For this review, take the finished solid that the model builds, in its own axes (mm). Coordinates: 2 decimals unless noted, no trailing zeros. Write each loop counter-clockwise with the first axis right and the second up, starting at its lowest first coordinate (ties: lowest second). Pieces come first, ordered by that corner, then holes.
1) Insertion check: P1, Ø5, axis at x = 20.5, z = 13, coming from the +Y side; P2, Ø1.5, axis at x = 19.5, z = 4, coming from the -Y side; P3, Ø2, axis at y = 8.5, z = 6.5, coming from the +X side. Each pin has a flat end and moves straight along its axis. Give the tip position at first contact, or say it passes through.
2) To check wall thickness, follow line 1 along X through (y, z) = (-20, 22); line 2 along X through (y, z) = (21.5, 10.75); line 3 along Y through (x, z) = (-29, 15.75). State the ranges of each line that lie inside material, in increasing order.
3) We need section A-A on z = 18.75. Write out the cut boundary in (x, y).
from build123d import *

# Parameters (mm, degrees)
F1_DEPTH = 25


with BuildPart() as f1:
    # F0 (on Top) → F1 (new body)
    with BuildSketch(Plane.XY):
        Polygon((17.320508, 30), (-17.320508, 30), (-34.641016, 0), (-17.320508, -30), (17.320508, -30), (34.641016, 0), align=None)
    extrude(amount=F1_DEPTH)

    # F2 (on Front) → F3 (revolve, cut)
    with BuildSketch(Plane.XZ):
        Polygon((34.641016, 22.113249), (34.641016, 25), (29.641016, 25), align=None)
    revolve(axis=Axis((-0.115662, 0, 18.696133), (0.006201, 0, 0.999981)), mode=Mode.SUBTRACT)


solid = f1.part
Result:
1. P1: stops at y = 28.82
1. P2: stops at y = -27.52
1. P3: stops at x = 30.31
2. line 1: x = -23.09 to 23.09
2. line 2: x = -22.23 to 22.23
2. line 3: y = -9.77 to 9.77
3. outline: (-34.64, 0) - (-17.32, -30) - (17.32, -30) - (34.64, 0) - (17.32, 30) - (-17.32, 30) - close
